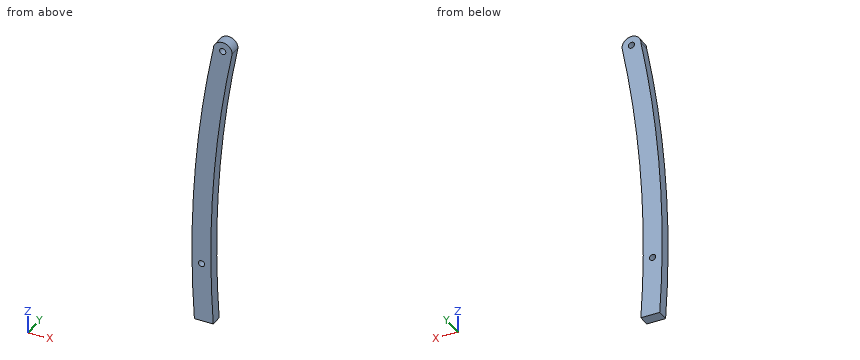
Autodesk Inventor part; units mm, degrees
ref_plane "YZ Plane" through (0, 0, 0) normal (1, 0, 0) x (0, 1, 0)
ref_plane "XZ Plane" through (0, 0, 0) normal (0, 1, 0) x (-1, 0, 0)
ref_plane "XY Plane" through (0, 0, 0) normal (0, 0, 1) x (1, 0, 0)
sketch "Sketch1" plane through (0, 0, 0) normal (0, 1, 0) x (-1, 0, 0)
  line L0 (0, 0) -> (0, -288.984) construction
  line L1 (5, 0) -> (5, -288.984)
  line L2 (-5, -288.984) -> (-5, 0)
  arc A0 (5, 0) -> (-5, 0) centre (0, 0) ccw
  arc A1 (-5, -288.984) -> (5, -288.984) centre (0, -288.984) ccw
  circle A2 centre (0, 0) radius 1.65
  circle A3 centre (0, -288.984) radius 1.65
  circle A4 centre (0, -231.585) radius 1.65
  arc A5 (-5, -231.585) -> (-5, 0) centre (-593.7207, -115.7925) ccw
  arc A6 (5, -231.585) -> (5, 0) centre (-583.7207, -115.7925) ccw
  circle A7 centre (11.23, -122.909) radius 1.65
  point P0 (0, -144.492)
  dimension "d0" = 3.3
  dimension "d1" = 3.3
  dimension "d2" = 10
  dimension "d3" = 288.984
  dimension "d14" = 3.3
  dimension "d15" = 231.585
  dimension "d18" = 600
  dimension "d19" = 600
  dimension "d20" = 3.3
  dimension "d21" = 122.909
extrude "Extrusion1" add sketch "Sketch1" along normal blind 6 contours L1 A1 L2 A5 | L1 A5 A6 | L1 A5 A0
sketch "Sketch2" plane through (0, 6, 0) normal (0, 1, 0) x (1, 0, 0)
  line L0 (-45.4801, 155.0502) -> (34.3076, 155.0502)
  line L1 (34.3076, 155.0502) -> (34.3076, -18.7731)
  line L2 (34.3076, -18.7731) -> (-45.4801, -18.7731)
  line L3 (-45.4801, -18.7731) -> (-45.4801, 155.0502)
  line L4 (-115.905, 316.254) -> (136.0777, 316.254)
  line L5 (136.0777, 316.254) -> (136.0777, -116.4724)
  line L6 (136.0777, -116.4724) -> (-115.905, -116.4724)
  line L7 (-115.905, -116.4724) -> (-115.905, 316.254)
  point P0 (0, 0)
extrude "Extrusion2" cut sketch "Sketch2" against normal blind 10
properties part number "Part_7_p1"
Verification items for the finished model (mm, model axes). Coordinates: 2 decimals unless noted, no trailing zeros. Order: outer loops, then holes, each group sorted by start corner. A loop starts at its lowest first (then second) coordinate and runs counter-clockwise, first axis right, second up.
1. Sectioned sample at B-B, the plane y = 3.15. Record the cut outline in (x, z).
Results found:
outline: (-14.99, -155.05) - (-4.99, -155.05) arc R600 cw to (5, 0) arc R5 ccw to (-5, 0) arc R600 ccw to start; hole circle Ø3.3 at (-11.23, -122.91); hole circle Ø3.3 at (0, 0)
2. Sectioned sample at C-C, the plane x = -11.23. Record the cut outline in (y, z).
Results found:
outline: (0, -155.05) - (6, -155.05) - (6, -124.56) - (0, -124.56) - close; (0, -121.26) - (6, -121.26) - (6, -38.12) - (0, -38.12) - close
3. Sectioned sample at D-D, the plane z = -50.5. Record the cut outline in (x, y), and give its area (3 significant figures).
Results found:
outline: (-12.72, 0) - (-2.72, 0) - (-2.72, 6) - (-12.72, 6) - close
area: 60.0 mm2
4. Sectioned sample at A-A, the plane x = 0. Record the cut outline in (y, z), and give its area (3 significant figures).
Results found:
outline: (0, -29.21) - (6, -29.21) - (6, -1.65) - (0, -1.65) - close; (0, 1.65) - (6, 1.65) - (6, 5) - (0, 5) - close
area: 185 mm2
5. Scan lines: line 1 (X direction, y = 2.6, z = -60.5); line 2 (X direction, y = 0.35, z = -75). Record each from-to range of solid material in increasing order.
Results found:
line 1: x = -13.73 to -3.73
line 2: x = -14.89 to -4.89
